The listing builds one solid part. Answer for the finished solid, in the listing's coordinates (mm). Face numbers are marked on the shaded views. A direction names the side the tool comes from. Round coordinates to 2 decimals unless told otherwise and drop trailing zeros. Write each loop counter-clockwise with the first axis right and the second up, starting at its lowest first coordinate (ties: lowest second). Pieces come first, ordered by that corner, then holes.
(1) Each of these flat-tipped pins is pushed along its axis until it touches: pin 1 Ø1.2 at (y, z) = (-1, -1) entering from -X; pin 2 Ø1.6 at (x, z) = (0, 0) entering from +Y; pin 3 Ø1 at (x, z) = (-7.5, 0) entering from -Y; pin 4 Ø1.3 at (x, y) = (-2, 0) entering from +Z. Where does it stop, or does it pass through?
(2) For the marked faces 1, 2 and 3, determine the directions among +Z, -Z, +X, -X, +Y, -Y from which every point of the face is accessible in a straight line to the end or side of a thin tool.
(3) A cutting plane is placed at C-C, the plane z = 0.8. Give the vertices of the cut face in (x, y).
(4) A cutting plane is placed at A-A, the plane y = 0. Give the vertices of the cut face in (x, z), and give its area (3 significant figures).
(5) Find the intervals of material crossed by probe 1 along Y at (x, z) = (-8.25, 0); probe 2 along Y at (x, z) = (0, 1.7); probe 3 along Z at (x, y) = (-7.5, -3.55), in increasing order.
(6) The mould has two halves that part along Z. Classify the marked faces 4, 5, 6 and 7: +Z half, -Z half, draft (parallel to the pull), parting line (faces both ways), or undercut.
(7) A cutting plane is placed at D-D, the plane x = 0. Give the vertices of the cut face in (y, z).
(8) A cutting plane is placed at B-B, the plane x = -7.5. Give the vertices of the cut face in (y, z).
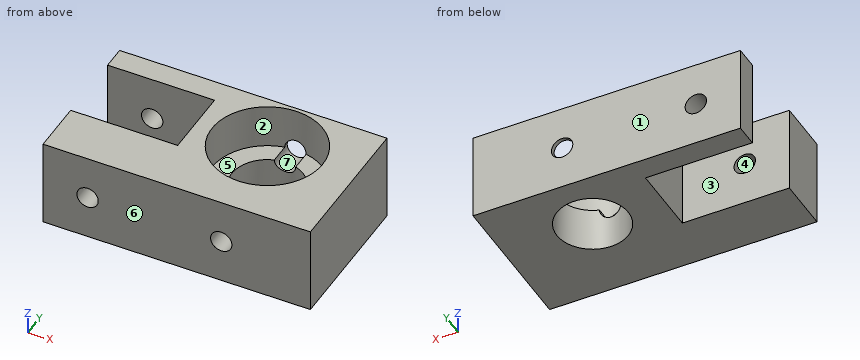
from build123d import *

# Parameters (mm, degrees)
SKETCH_1_W          = 20
SKETCH_1_H          = 10
SKETCH_1_R          = 3.1
EXTRUDE_1_DEPTH     = 2.5
SKETCH_2_W          = 20
SKETCH_2_H          = 10
EXTRUDE_2_DEPTH     = 2.5
SKETCH_3_R          = 0.6
CUT_EXTRUDE_1_DEPTH = 15.361406616
SKETCH_4_W          = 6
SKETCH_4_H          = 4
CUT_EXTRUDE_2_DEPTH = 13.247448796
SKETCH_5_R          = 2
CUT_EXTRUDE_3_DEPTH = 13.247448755
SKETCH_6_W          = 20
SKETCH_6_H          = 1.7
CUT_EXTRUDE_4_DEPTH = 13.247448796
SKETCH_7_W          = 5
SKETCH_7_H          = 8.3
CUT_EXTRUDE_5_DEPTH = 13.247448796


with BuildPart() as part:
    # 草图1 → 凸台-拉伸1 (new body)
    with BuildSketch(Plane.XY):
        Rectangle(SKETCH_1_W, SKETCH_1_H)
        Circle(SKETCH_1_R, mode=Mode.SUBTRACT)
    extrude(amount=EXTRUDE_1_DEPTH)

    # 草图2 → 凸台-拉伸2 (add)
    with BuildSketch(Plane(origin=(0, 0, 0), x_dir=(-1, 0, 0), z_dir=(0, 0, -1))):
        Rectangle(SKETCH_2_W, SKETCH_2_H)
    extrude(amount=EXTRUDE_2_DEPTH)

    # 草图3 → 切除-拉伸1 (cut, through all)
    with BuildSketch(Plane.XZ.offset(5)):
        with Locations((-7.5, 0)):
            Circle(SKETCH_3_R)
        Circle(SKETCH_3_R)
    extrude(amount=-CUT_EXTRUDE_1_DEPTH, mode=Mode.SUBTRACT)

    # 草图4 → 切除-拉伸2 (cut, through all)
    with BuildSketch(Plane(origin=(0, 0, -2.5), x_dir=(-1, 0, 0), z_dir=(0, 0, -1))):
        with Locations((7, 0)):
            Rectangle(SKETCH_4_W, SKETCH_4_H)
    extrude(amount=-CUT_EXTRUDE_2_DEPTH, mode=Mode.SUBTRACT)

    # 草图5 → 切除-拉伸3 (cut, through all)
    with BuildSketch(Plane.XY.offset(2.5)):
        Circle(SKETCH_5_R)
    extrude(amount=-CUT_EXTRUDE_3_DEPTH, mode=Mode.SUBTRACT)

    # 草图6 → 切除-拉伸4 (cut, through all)
    with BuildSketch(Plane.XY.offset(2.5)):
        with Locations((0, 4.15)):
            Rectangle(SKETCH_6_W, SKETCH_6_H)
    extrude(amount=-CUT_EXTRUDE_4_DEPTH, mode=Mode.SUBTRACT)

    # 草图7 → 切除-拉伸5 (cut, through all)
    with BuildSketch(Plane.XY.offset(2.5)):
        with Locations((7.5, -0.85)):
            Rectangle(SKETCH_7_W, SKETCH_7_H)
    extrude(amount=-CUT_EXTRUDE_5_DEPTH, mode=Mode.SUBTRACT)


solid = part.part
Solutions:
1. pin 1: stops at x = -4
1. pin 2: stops at y = 3.3
1. pin 3: passes through
1. pin 4: stops at z = 0
2. face 1: +Z, -Z, +X, -X, +Y
2. face 2: +Z
2. face 3: +Z, -Z, -X
3. outline: (-10, -5) - (5, -5) - (5, 3.3) - (-10, 3.3) - (-10, 2) - (-4, 2) - (-4, -2) - (-10, -2) - close; hole circle Ø6.2 at (0, 0)
4. outline: (-4, -2.5) - (-2, -2.5) - (-2, 0) - (-3.1, 0) - (-3.1, 2.5) - (-4, 2.5) - close; (2, -2.5) - (5, -2.5) - (5, 2.5) - (3.1, 2.5) - (3.1, 0) - (2, 0) - close
4. area: 19.5 mm2
5. probe 1: y = -5 to -2, 2 to 3.3
5. probe 2: y = -5 to -3.1, 3.1 to 3.3
5. probe 3: z = -2.5 to -0.6, 0.6 to 2.5
6. face 4: undercut
6. face 5: +Z half
6. face 6: draft
6. face 7: undercut
7. outline: (-5, -2.5) - (-2, -2.5) - (-2, -0.6) - (-5, -0.6) - close; (-5, 0.6) - (-3.1, 0.6) - (-3.1, 2.5) - (-5, 2.5) - close; (2, -2.5) - (3.3, -2.5) - (3.3, -0.6) - (2, -0.6) - close; (3.1, 0.6) - (3.3, 0.6) - (3.3, 2.5) - (3.1, 2.5) - close
8. outline: (-5, -2.5) - (-2, -2.5) - (-2, -0.6) - (-5, -0.6) - close; (-5, 0.6) - (-2, 0.6) - (-2, 2.5) - (-5, 2.5) - close; (2, -2.5) - (3.3, -2.5) - (3.3, -0.6) - (2, -0.6) - close; (2, 0.6) - (3.3, 0.6) - (3.3, 2.5) - (2, 2.5) - close
